```python
from build123d import *

# Parameters (mm, degrees)
F0_R      = 19.05
F1_DEPTH  = 63.5
F3_R      = 12.7
F4_DEPTH  = 50.8
F6_DEPTH  = 43.942
F7_R      = 3.125
F8_DEPTH  = 53.594
F10_DEPTH = 5.5


with BuildPart() as f1:
    # F0 (on Top) → F1 (new body)
    with BuildSketch(Plane.XY):
        Circle(F0_R)
    extrude(amount=F1_DEPTH)

    # F3 (on face) → F4 (cut)
    with BuildSketch(Plane.XY.offset(63.5)):
        Circle(F3_R)
    extrude(amount=-F4_DEPTH, mode=Mode.SUBTRACT)

    # F5 (on face) → F6 (cut)
    with BuildSketch(Plane.XY.offset(63.5)):
        Polygon((0, 38.1), (0, 0), (2.54, 38.1), align=None)
        Polygon((-14.580239, 35.19981), (0, 0), (-12.233585, 36.171826), align=None)
        Polygon((-26.940768, 26.940768), (0, 0), (-25.144717, 28.73682), align=None)
        Polygon((-35.19981, 14.580239), (0, 0), (-34.227794, 16.926893), align=None)
        Polygon((-38.1, 0), (0, 0), (-38.1, 2.54), align=None)
        Polygon((-35.19981, -14.580239), (0, 0), (-36.171826, -12.233585), align=None)
        Polygon((-26.940768, -26.940768), (0, 0), (-28.73682, -25.144717), align=None)
        Polygon((-14.580239, -35.19981), (0, 0), (-16.926893, -34.227794), align=None)
        Polygon((0, -38.1), (0, 0), (-2.54, -38.1), align=None)
        Polygon((14.580239, -35.19981), (0, 0), (12.233585, -36.171826), align=None)
        Polygon((26.940768, -26.940768), (0, 0), (25.144717, -28.73682), align=None)
        Polygon((35.19981, -14.580239), (0, 0), (34.227794, -16.926893), align=None)
        Polygon((38.1, 0), (0, 0), (38.1, -2.54), align=None)
        Polygon((35.19981, 14.580239), (0, 0), (36.171826, 12.233585), align=None)
        Polygon((26.940768, 26.940768), (0, 0), (28.73682, 25.144717), align=None)
        Polygon((14.580239, 35.19981), (0, 0), (16.926893, 34.227794), align=None)
    extrude(amount=-F6_DEPTH, mode=Mode.SUBTRACT)

    # F7 (on face) → F8 (cut)
    with BuildSketch(Plane.XY.offset(12.7)):
        Circle(F7_R)
    extrude(amount=-F8_DEPTH, mode=Mode.SUBTRACT)

    # F9 (on face) → F10 (cut)
    with BuildSketch(Plane.XY.offset(12.7)):
        Polygon((0.699814, -6.341222), (5.841566, -2.564554), (5.141752, 3.776668), (-0.699814, 6.341222), (-5.841566, 2.564554), (-5.141752, -3.776668), align=None)
    extrude(amount=-F10_DEPTH, mode=Mode.SUBTRACT)

    # F11 (on Right) → F12 (revolve, cut)
    with BuildSketch(Plane.YZ):
        Polygon((-16.030312, 63.901735), (-19.12548, 63.898501), (-19.12548, 20.142671), align=None)
    revolve(axis=Axis((0, 0, -11.778668), (0, 0, -1)), mode=Mode.SUBTRACT)


solid = f1.part
```
The listing builds one solid part. Answer for the finished solid, in the listing's coordinates (mm). A direction names the side the tool comes from. Give positions to 0.01 mm unless a question says otherwise; leave off trailing zeros. Write each loop counter-clockwise with the first axis right and the second up, starting at its lowest first coordinate (ties: lowest second). Pieces come first, ordered by that corner, then holes. Notation, with made-up numbers: (82.5, 39) -> (128.5, 39) arc R27 ccw to (128.5, 63) -> close; hole circle Ø3 at (31, 73.5). An arc over 180 degrees is marked (long way). Use one line per item in the form item = value.
1) Section B-B on z = 38 is taken. Count the separate pieces of the cut face and the enclosed holes in it, plus the area to 3 significant figures.
Result:
separate_pieces = 16
enclosed_holes = 0
area = 412 mm²
2) Each of these flat-tipped pins is pushed along its axis until it touches: P1, Ø1.4, axis at x = 0.5, y = 15.5, coming from the +Z side; P2, Ø1, axis at x = -1.5, z = 55.5, coming from the +Y side; P3, Ø7.5, axis at x = -6, y = 6, coming from the +Z side; P4, Ø1.9, axis at x = -15.5, z = 51, coming from the +Y side. Where does it stop, or does it pass through?
Result:
P1 = 63.5
P2 = 16.61
P3 = 12.7
P4 = 8.69
3) Straight lines are drawn through the part: probe 1 along Y at (x, z) = (0, 3.25) (3 decimals); probe 2 along Z at (x, y) = (6.5, 2); probe 3 along Z at (x, y) = (-4, -1). For each, find the intervals that lie inside material, in ascending order.
Result:
probe_1 = -19.05 to -3.125, 3.125 to 19.05
probe_2 = 0 to 12.7
probe_3 = 0 to 7.2
4) A tool of negligible diameter and unlimited length cuts with its end or side. For faces 1 (the flat face through (-15, 1, 42)), 2 (the flat face through (0, -15, 42)), 3 (the flat face through (3.235, -4.479, 9.988)), from which of +Z, -Z, +X, -X, +Y, -Y can it reach the whole face along a straight path? Write none if from no direction.
Result:
face_1 = +Z, -X
face_2 = +Z, -Y
face_3 = +Z
5) Section A-A on z = 16.5 is taken. Write down the section's boundary in (x, y).
Result:
outline = circle Ø38.1 at (0, 0); hole circle Ø25.4 at (0, 0)
6) For a pull along Y with two mould halves and no side action, classify faces 4 (the flat face through (5.822, 14.056, 41.837)), 5 (the flat face through (-11, 11, 42)), 6 (the cylindrical face through (-2.48, 18.888, 10.456)), 7 (the flat face through (0.5, 15.9, 19.558)) as +Y half, -Y half, draft (parallel to the pull), parting line (faces both ways), or undercut.
Result:
face_4 = undercut
face_5 = undercut
face_6 = parting line
face_7 = draft
